Verification items for the finished model (mm, model axes). A direction names the side the tool comes from. Give positions to 0.01 mm unless a question says otherwise; leave off trailing zeros. Write each loop counter-clockwise with the first axis right and the second up, starting at its lowest first coordinate (ties: lowest second). Pieces come first, ordered by that corner, then holes. Notation, with made-up numbers: (41, 72) - (63, 72) arc R31 cw to (63, 97) - close; hole circle Ø3 at (31, 41). An arc over 180 degrees is marked (long way). Put each result on its own line as item: value.
from build123d import *

# Parameters (mm, degrees)
SKETCH2_W           = 8
SKETCH2_H           = 50
SKETCH2_R           = 2.25
BOSS_EXTRUDE1_DEPTH = 60
SKETCH3_R           = 2
BOSS_EXTRUDE2_DEPTH = 5


with BuildPart() as part:
    # Sketch2 → Boss-Extrude1 (new body)
    # profile 1 of 4: a face of its own
    with BuildSketch(Plane(origin=(0, 0, 0), x_dir=(1, 0, 0), z_dir=(0, 1, 0))):
        with Locations((-19.731065886, 6.378485879)):
            Rectangle(SKETCH2_W, SKETCH2_H)
        with Locations((-19.731065886, 20.878485879)):
            Circle(SKETCH2_R, mode=Mode.SUBTRACT)
        with Locations((-19.731065886, 12.878485879)):
            Circle(SKETCH2_R, mode=Mode.SUBTRACT)
        with Locations((-19.731065886, 4.878485879)):
            Circle(SKETCH2_R, mode=Mode.SUBTRACT)
    # profile 2 of 4: a face of its own
    with BuildSketch(Plane(origin=(0, 0, 0), x_dir=(1, 0, 0), z_dir=(0, 1, 0))):
        with Locations((-19.731065886, 20.878485879)):
            Circle(SKETCH2_R)
    # profile 3 of 4: a face of its own
    with BuildSketch(Plane(origin=(0, 0, 0), x_dir=(1, 0, 0), z_dir=(0, 1, 0))):
        with Locations((-19.731065886, 12.878485879)):
            Circle(SKETCH2_R)
    # profile 4 of 4: a face of its own
    with BuildSketch(Plane(origin=(0, 0, 0), x_dir=(1, 0, 0), z_dir=(0, 1, 0))):
        with Locations((-19.731065886, 4.878485879)):
            Circle(SKETCH2_R)
    extrude(amount=BOSS_EXTRUDE1_DEPTH)

    # Sketch3 → Boss-Extrude2 (add)
    with BuildSketch(Plane.XZ):
        with Locations(Location((-19.731065886, -4.878485879, 0), (0, 0, 90))):
            Circle(SKETCH3_R)
        with Locations(Location((-19.731065886, -12.878485879, 0), (0, 0, 90))):
            Circle(SKETCH3_R)
        with Locations(Location((-19.731065886, -20.878485879, 0), (0, 0, 90))):
            Circle(SKETCH3_R)
    extrude(amount=BOSS_EXTRUDE2_DEPTH)


solid = part.part
Q1. Section check C-C, the plane z = -6. Record the cut outline in (x, y), plus the area to 3 significant figures.
Answers follow:
outline: (-23.73, 0) - (-21.39, 0) - (-21.39, -5) - (-18.08, -5) - (-18.08, 0) - (-15.73, 0) - (-15.73, 60) - (-23.73, 60) - close
area: 497 mm2
Q2. Release check for a two-part mould opening along Z. For faces 3 (the face through (-20, -5, -21)), 4 (the face through (-20, 30, 18.622)), 5 (the face through (-19.819, -2.465, -14.877)) record: released by +Z, released by -Z, zero draft, split by the parting line, or undercut.
Answers follow:
face 3: zero draft
face 4: released by +Z
face 5: undercut
Q3. Scan line: line 1 along Y through (x, z) = (-18.5, -7.5). Record every from-to range of solid material in increasing order.
Answers follow:
line 1: y = 0 to 60
Q4. Set-up check for faces 1 (the face through (-20.33, -2.46, -2.97)), 2 (the face through (-15.731, 30, -6)): record each of +Z, -Z, +X, -X, +Y, -Y from which the full face is reachable in a straight line by a thin tool's end or side.
Answers follow:
face 1: -Y
face 2: +Z, -Z, +X, +Y, -Y
Q5. Section check D-D, the plane z = 3. Record the cut outline in (x, y).
Answers follow:
outline: (-23.73, 0) - (-15.73, 0) - (-15.73, 60) - (-23.73, 60) - close
Q6. Section check A-A, the plane z = -21. Record the cut outline in (x, y).
Answers follow:
outline: (-23.73, 0) - (-21.73, 0) - (-21.73, -5) - (-17.73, -5) - (-17.73, 0) - (-15.73, 0) - (-15.73, 60) - (-23.73, 60) - close
Q7. Section check B-B, the plane x = -21. Record the cut outline in (y, z), plus the area to 3 significant figures.
Answers follow:
outline: (-5, -22.42) - (0, -22.42) - (0, -31.38) - (60, -31.38) - (60, 18.62) - (0, 18.62) - (0, -3.33) - (-5, -3.33) - (-5, -6.42) - (0, -6.42) - (0, -11.33) - (-5, -11.33) - (-5, -14.42) - (0, -14.42) - (0, -19.33) - (-5, -19.33) - close
area: 3,050 mm2
